Part model, mm, in its own coordinate system. A direction names the side the tool comes from. Give positions to 0.01 mm unless a question says otherwise; leave off trailing zeros. Loops run counter-clockwise (first coordinate to the right, second up) from the corner with the lowest first, then second, coordinate; pieces in that order, holes last. Notation, with made-up numbers: (58.25, 44) -> (64.25, 44) arc R20 ccw to (64.25, 64) -> close; hole circle Ø7 at (49, 42). An arc over 180 degrees is marked (long way). Write item = value, one per line.
from build123d import *

# Parameters (mm, degrees)
F0_W      = 600
F0_H      = 600
F1_DEPTH  = 20
F1_FACE_W = 600
F1_FACE_H = 600
F5_T      = -20


with BuildPart() as f1:
    # F0 (on Top) → F1 (new body)
    with BuildSketch(Plane.XY):
        Rectangle(F0_W, F0_H)
    extrude(amount=F1_DEPTH)

    # F1_face (on face) → F4 section 0
    with BuildSketch(Plane.XY.offset(20), mode=Mode.PRIVATE) as f4_s0:
        Rectangle(F1_FACE_W, F1_FACE_H)
    loft([f4_s0.sketch, Vertex(0, 0, 520)])

    # F5
    f5_openings = [f1.faces().sort_by_distance(p)[0] for p in [
        (0, 0, 0),
    ]]
    offset(amount=F5_T, openings=f5_openings)


solid = f1.part
1) Drop flat-ended pins along their axis: P1, Ø2, axis at x = 21.5, z = 467, coming from the -Y side; P2, Ø2, axis at x = 204.5, y = 108.5, coming from the +Z side; P3, Ø1.5, axis at x = 198, z = 57.5, coming from the -Y side. Give the stop position or say it passes through.
Resolved:
P1 = -32.4
P2 = 180.83
P3 = -277.95
2) Slice it at D-D, the plane z = 141. List the corners of the cut face in (x, y), and give its area (3 significant figures).
Resolved:
outline = (-227.4, -227.4) -> (227.4, -227.4) -> (227.4, 227.4) -> (-227.4, 227.4) -> close; hole (-204.08, -204.08) -> (204.08, -204.08) -> (204.08, 204.08) -> (-204.08, 204.08) -> close
area = 40,300 mm²
3) Drill centre lines: line 1 along X through (y, z) = (9.5, 420); line 2 along X through (y, z) = (62.5, 338); line 3 along Y through (x, z) = (-1, 280). Where is each one in solid material? Low to high. Write a range as [from, to].
Resolved:
line_1 = [-60, -36.68], [36.68, 60]
line_2 = [-109.2, -85.88], [85.88, 109.2]
line_3 = [-144, -120.68], [120.68, 144]
4) Slice it at B-B, the plane x = -60. List the corners of the cut face in (y, z), and give its area (3 significant figures).
Resolved:
outline = (-300, 0) -> (-280, 0) -> (-280, 14.46) -> (-60, 381.13) -> (60, 381.13) -> (280, 14.46) -> (280, 0) -> (300, 0) -> (300, 20) -> (60, 420) -> (-60, 420) -> (-300, 20) -> close
area = 23,200 mm²
5) Pull direction Y, two halves, no side cores. Call faces 3 (the face through (169.15, -3.92, 199.21)), 4 (the face through (-4, 300, 10)), 5 (the face through (-300, -4, 10)): pulls with the +Y half, pulls with the -Y half, needs draft (parallel to the pull), parting line crosses it, or undercut.
Resolved:
face_3 = undercut
face_4 = pulls with the +Y half
face_5 = needs draft
6) Slice it at C-C, the plane y = -67. List the corners of the cut face in (x, z), and give its area (3 significant figures).
Resolved:
outline = (-300, 0) -> (-280, 0) -> (-280, 14.46) -> (-67, 369.46) -> (67, 369.46) -> (280, 14.46) -> (280, 0) -> (300, 0) -> (300, 20) -> (67, 408.33) -> (-67, 408.33) -> (-300, 20) -> close
area = 23,200 mm²
7) Which spindle directions (+Z, -Z, +X, -X, +Y, -Y) get a long thin tool onto all of the face, cutting with end or side? Do faces 1 (the face through (-181.233, 4.2, 217.944)), 2 (the face through (3.92, 169.15, 199.21)). Say none if no direction does.
Resolved:
face_1 = +Z, -X, +Y, -Y
face_2 = -Z
8) Slice it at A-A, the plane z = 343.5. List the corners of the cut face in (x, y).
Resolved:
outline = (-105.9, -105.9) -> (105.9, -105.9) -> (105.9, 105.9) -> (-105.9, 105.9) -> close; hole (-82.58, -82.58) -> (82.58, -82.58) -> (82.58, 82.58) -> (-82.58, 82.58) -> close
